```python
from build123d import *

# Parameters (mm, degrees)
F0_R     = 5
F0_R_2   = 4
F1_DEPTH = 8.5


with BuildPart() as f1:
    # F0 (on Top) → F1 (new body, symmetric)
    with BuildSketch(Plane.XY):
        with BuildLine():
            ThreePointArc((-23.748692, 79.59965), (-47.98176, 80.727368), (-55.475573, 57.654524))
            Line((-55.475573, 57.654524), (-18.871129, -46.624236))
            ThreePointArc((-18.871129, -46.624236), (-4.440782, -59.500755), (14.142136, -54.142136))
            Line((14.142136, -54.142136), (54.142136, -14.142136))
            ThreePointArc((54.142136, -14.142136), (59.980964, 0.872388), (52.855752, 15.320889))
            Line((52.855752, 15.320889), (-23.748692, 79.59965))
        make_face()
        with Locations((0, -40)):
            Circle(F0_R, mode=Mode.SUBTRACT)
        with BuildLine():
            Line((4.057651, 10.578103), (15.310351, 1.135966))
            ThreePointArc((15.310351, 1.135966), (16.379133, -1.031309), (15.503309, -3.283488))
            Line((15.503309, -3.283488), (9.627566, -9.159231))
            ThreePointArc((9.627566, -9.159231), (6.840128, -9.963024), (4.675576, -8.031546))
            Line((4.675576, -8.031546), (-0.701381, 7.286334))
            ThreePointArc((-0.701381, 7.286334), (0.422691, 10.74726), (4.057651, 10.578103))
        make_face(mode=Mode.SUBTRACT)
        with Locations((40, 0)):
            Circle(F0_R_2, mode=Mode.SUBTRACT)
        with Locations((-36.604444, 64.278761)):
            Circle(F0_R_2, mode=Mode.SUBTRACT)
    extrude(amount=F1_DEPTH, both=True)


solid = f1.part
```
Geometry: final body of the model. Coordinates: model frame, mm. A direction names the side the tool comes from. Round coordinates to 2 decimals unless told otherwise and drop trailing zeros. Write each loop counter-clockwise with the first axis right and the second up, starting at its lowest first coordinate (ties: lowest second). Pieces come first, ordered by that corner, then holes. Notation, with made-up numbers: (49.25, 33) -> (86.25, 33) arc R21 ccw to (86.25, 40) -> close; hole circle Ø9 at (6, 13.25). An arc over 180 degrees is marked (long way). Use CSV: the item, a comma, the result in double quotes. Start each with the question number.
Q1. Reachability of faces 5 (the face through (6.88, -9.97, 0.12)), 6 (the face through (33.862, -34.422, 0.119)) from +Z, -Z, +X, -X, +Y, -Y: full face, straight path, thin tool, end or side. Return the list, or none.
Q2. Pull-direction query (Y, two-part tool) for faces 1 (the face through (1, 13, -8.5)), 2 (the face through (16.377, -0.997, 0.119)), 3 (the face through (-37.43, 6.25, 0.12)), 4 (the face through (15.1, 47, 0.1)); classes: pulls with the +Y half, pulls with the -Y half, needs draft (parallel to the pull), parting line crosses it, or undercut.
Q3. Section B-B (x = 40). Return loops of the section in (y, z), plus the area to 3 significant figures.
Q4. Section C-C (z = -4.25). Return loops of the section in (x, y).
Q5. First-contact query: pin 1 Ø1.5 at (y, z) = (-13.5, 2.5) entering from -X; pin 2 Ø1.5 at (y, z) = (11, 2.5) entering from -X; pin 3 Ø6.5 at (x, y) = (40, 0) entering from +Z; pin 4 Ø4 at (x, z) = (-27, 6.5) entering from +Y. Flat tips, straight axial feed; report the tip coordinate or a pass-through.
Q6. Section A-A (y = -40). Return loops of the section in (x, z), plus the area to 3 significant figures.
Q7. Section D-D (y = -24.5). Return loops of the section in (x, z), plus the area to 3 significant figures.
Q8. Line query: L1, parallel to X at y = -3, z = 3.25; L2, parallel to X at y = 9, z = 2.5; L3, parallel to Y at x = 40, z = 0.75. Output: solid intervals per line, ascending.
Result sheet:
1,face 5,"+Z, -Z"
1,face 6,"+Z, -Z, +X, -Y"
2,face 1,"needs draft"
2,face 2,"undercut"
2,face 3,"pulls with the -Y half"
2,face 4,"pulls with the +Y half"
3,outline,"(-28.28, -8.5) -> (-4, -8.5) -> (-4, 8.5) -> (-28.28, 8.5) -> close; (4, -8.5) -> (26.11, -8.5) -> (26.11, 8.5) -> (4, 8.5) -> close"
3,area,"789 mm²"
4,outline,"(-55.48, 57.65) -> (-18.87, -46.62) arc R20 ccw to (14.14, -54.14) -> (54.14, -14.14) arc R20 ccw to (52.86, 15.32) -> (-23.75, 79.6) arc R20 ccw to start; hole circle Ø8 at (-36.6, 64.28); hole circle Ø10 at (0, -40); hole (-0.7, 7.29) -> (4.68, -8.03) arc R3 ccw to (9.63, -9.16) -> (15.5, -3.28) arc R3 ccw to (15.31, 1.14) -> (4.06, 10.58) arc R3 ccw to start; hole circle Ø8 at (40, 0)"
5,pin 1,"x = -30.76"
5,pin 2,"x = -39.36"
5,pin 3,"through"
5,pin 4,"y = 82.78"
6,outline,"(-21.2, -8.5) -> (-5, -8.5) -> (-5, 8.5) -> (-21.2, 8.5) -> close; (5, -8.5) -> (28.28, -8.5) -> (28.28, 8.5) -> (5, 8.5) -> close"
6,area,"671 mm²"
7,outline,"(-26.64, -8.5) -> (43.78, -8.5) -> (43.78, 8.5) -> (-26.64, 8.5) -> close"
7,area,"1,200 mm²"
8,L1,"-34.18 to 2.91, 15.75 to 37.35, 42.65 to 59.77"
8,L2,"-38.4 to -0.78, 5.94 to 57.86"
8,L3,"-28.28 to -4, 4 to 26.11"
